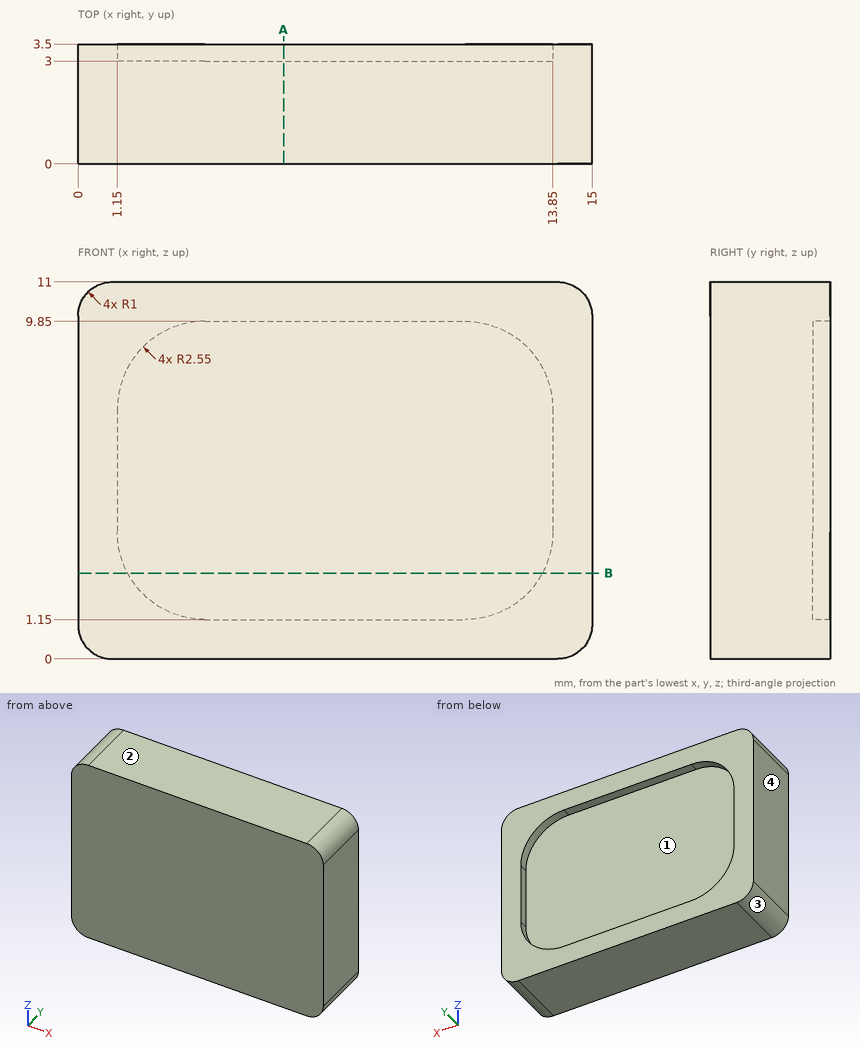
Can you work these out from the drawing? Everything is in mm from the part's minimum corner. Give positions to 0.01 mm unless a question says otherwise; leave off trailing zeros. Loops run counter-clockwise (first coordinate to the right, second up) from the corner with the lowest first, then second, coordinate; pieces in that order, holes last. Notation, with made-up numbers: (81, -35.75) -> (140, -35.75) arc R13 ccw to (140, -15.75) -> close; hole circle Ø2 at (19, 2.25). An arc over 180 degrees is marked (long way). Return JSON: item names as keys, results as strings.
Q1. I need wall thicknesses on probe 1 along X at (y, z) = (3.3, 6.75); probe 2 along Y at (x, z) = (10, 5); probe 3 along X at (y, z) = (3.25, 2.25). Which ranges of each line are inside material? Lowest first, please.
Checks:
{"probe 1": "x = 0 to 1.15, 13.85 to 15", "probe 2": "y = 0 to 3", "probe 3": "x = 0 to 1.6, 13.4 to 15"}
Q2. For pin 1 Ø1.5 at (y, z) = (1, 1.5) entering from -X; pin 2 Ø1.5 at (x, z) = (12, 3.5) entering from +Y, each with a flat end and sliding along its axis, tell me the tip position at first contact or that it passes through.
Checks:
{"pin 1": "stops at x = 0", "pin 2": "stops at y = 3"}
Q3. I want a section at B-B, the plane z = 2.5. List the corners of the cut face in (x, y) for me.
Checks:
{"outline": "(0, 0) -> (15, 0) -> (15, 3.5) -> (13.55, 3.5) -> (13.55, 3) -> (1.45, 3) -> (1.45, 3.5) -> (0, 3.5) -> close"}
Q4. We'd pull the mould along Z, two halves only. Please class the marked faces 1, 2, 3 and 4: released by +Z, released by -Z, zero draft, split by the parting line, or undercut.
Checks:
{"face 1": "undercut", "face 2": "released by +Z", "face 3": "released by -Z", "face 4": "zero draft"}
Q5. I want a section at A-A, the plane x = 6. List the corners of the cut face in (y, z) for me, then the cut area to 4 significant figures.
Checks:
{"outline": "(0, 0) -> (3.5, 0) -> (3.5, 1.15) -> (3, 1.15) -> (3, 9.85) -> (3.5, 9.85) -> (3.5, 11) -> (0, 11) -> close", "area": "34.15 mm2"}
